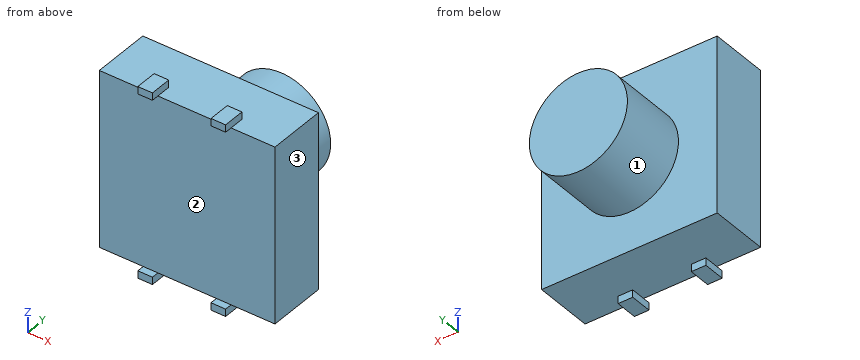
Autodesk Inventor part; units mm, degrees
ref_plane "YZ Plane" through (0, 0, 0) normal (1, 0, 0) x (0, 1, 0)
ref_plane "XZ Plane" through (0, 0, 0) normal (0, 1, 0) x (-1, 0, 0)
sketch "Sketch1" plane through (0, 0, 0) normal (0, 1, 0) x (-1, 0, 0)
  line L0 (-6, 6) -> (6, 6)
  line L1 (6, 6) -> (6, -6)
  line L2 (6, -6) -> (-6, -6)
  line L3 (-6, -6) -> (-6, 6)
  line L4 (-6, 6) -> (6, -6) construction
  line L5 (6, 6) -> (-6, -6) construction
  point P0 (0, 0)
  dimension "d0" = 12
  dimension "d1" = 12
extrude "Extrusion1" add sketch "Sketch1" along normal blind 4
sketch "Sketch2" plane through (0, 4, 0) normal (0, 1, 0) x (1, 0, 0)
  circle A0 centre (0, 0) radius 3.35
  dimension "d4" = 6.7
extrude "Extrusion2" add sketch "Sketch2" along normal blind 4.7
sketch "Sketch3" plane through (-6, 0, 6) normal (0, 0, 1) x (1, 0, 0)
  line L0 (3, 1) -> (4, 1)
  line L1 (4, 1) -> (4, -0.5)
  line L2 (12, 0) -> (0, 0)
  line L3 (4, -0.5) -> (3, -0.5)
  line L4 (3, -0.5) -> (3, 1)
  line L5 (0, 0) -> (0, 4)
  line L6 (6, 3.8576) -> (6, 0) construction
  line L7 (9, 1) -> (8, 1)
  line L8 (8, 1) -> (8, -0.5)
  line L9 (8, -0.5) -> (9, -0.5)
  line L10 (9, -0.5) -> (9, 1)
  dimension "d7" = 1
  dimension "d8" = 1
  dimension "d9" = 1.5
  dimension "d10" = 3
extrude "Extrusion3" add sketch "Sketch3" along normal blind 0.5
mirror "Mirror1" about plane through (0, 0, 0) normal (0, 0, 1) of "Extrusion3"
properties part number "Push_Button"
Geometry check sheet. Reference: the model listing, model coordinates, mm. Face numbers are marked on the shaded views. A direction names the side the tool comes from. Give positions to 0.01 mm unless a question says otherwise; leave off trailing zeros. Order: outer loops, then holes, each group sorted by start corner. A loop starts at its lowest first (then second) coordinate and runs counter-clockwise, first axis right, second up. Notation, with made-up numbers: (61, -29) - (115, -29) arc R27 cw to (115, 9) - close; hole circle Ø9 at (-7.5, 31). An arc over 180 degrees is marked (long way). Answer in a Markdown table with one row per item. Add a question column.
Q1. Cross-section at A-A, the plane z = 0. Enter the section's corners in (x, y), then the cut area to 3 significant figures.
Q2. Cross-section at B-B, the plane x = -1.5. Enter the section's corners in (y, z), then the cut area to 3 significant figures.
Q3. Cross-section at D-D, the plane x = 5. Enter the section's corners in (y, z).
Q4. Material ranges on probe 1 along Y at (x, z) = (1.75, 0.25); probe 2 along Y at (x, z) = (1, 4.25); probe 3 along Z at (x, y) = (-3.25, 0.25), recorded low to high. Write a range as from..to.
Q5. Tool access check on the marked faces 1, 2 and 3. Record the directions out of +Z, -Z, +X, -X, +Y, -Y that give a thin tool (end or side, any length) a straight path to the whole face; none if there is none.
Q6. Gauge pin test, flat ends, axial feed: pin 1 (3 mm diameter, centred on x = -4.5, z = -1, fed in from -Y); pin 2 (2 mm diameter, centred on x = 0.5, y = 1.5, fed in from -Z); pin 3 (5 mm diameter, centred on x = 3.5, z = 5, fed in from +Y). Record the tip position at first contact, or that the pin passes through.
Q7. Cross-section at C-C, the plane y = 6.5. Enter the section's corners in (x, z).
Check values:
| question | item | result |
|---|---|---|
| 1 | outline | (-6, 0) - (6, 0) - (6, 4) - (3.35, 4) - (3.35, 8.7) - (-3.35, 8.7) - (-3.35, 4) - (-6, 4) - close |
| 1 | area | 79.5 mm^2 |
| 2 | outline | (0, -6) - (4, -6) - (4, -3) - (8.7, -3) - (8.7, 3) - (4, 3) - (4, 6) - (0, 6) - close |
| 2 | area | 76.2 mm^2 |
| 3 | outline | (0, -6) - (4, -6) - (4, 6) - (0, 6) - close |
| 4 | probe 1 | y = 0..8.7 |
| 4 | probe 2 | y = 0..4 |
| 4 | probe 3 | z = -6..6 |
| 5 | face 1 | +Y |
| 5 | face 2 | +X, -X, -Y |
| 5 | face 3 | +Z, -Z, +X, +Y, -Y |
| 6 | pin 1 | stops at y = 0 |
| 6 | pin 2 | stops at z = -6 |
| 6 | pin 3 | stops at y = 4 |
| 7 | outline | circle Ø6.7 at (0, 0) |
